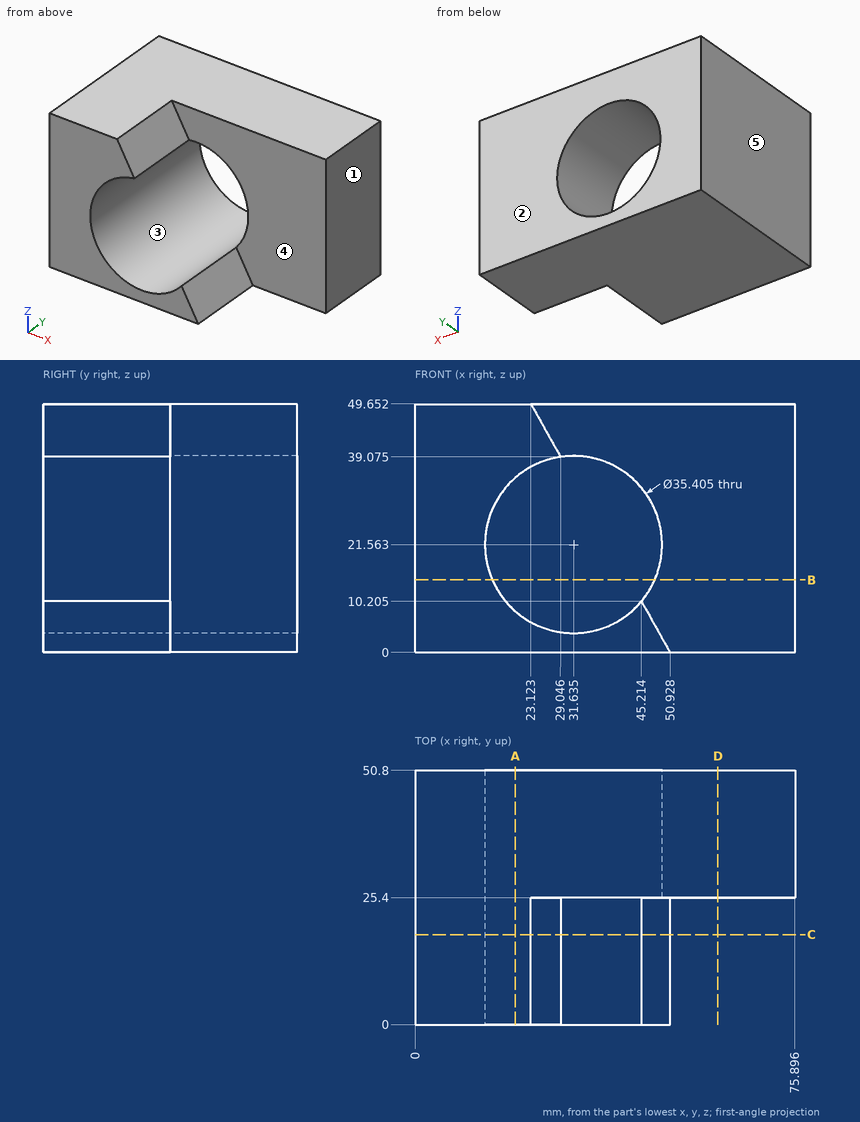
Verification items for this drawing (mm, ordinates from the low corner). A direction names the side the tool comes from. Coordinates: 2 decimals unless noted, no trailing zeros. Loops run counter-clockwise (first coordinate to the right, second up) from the corner with the lowest first, then second, coordinate; pieces in that order, holes last. Notation, with made-up numbers: (-9.75, 38) - (11.25, 38) arc R4 cw to (11.25, 44) - close; hole circle Ø10 at (46.25, -13.75). An arc over 180 degrees is marked (long way). Answer as a JSON object with one key per item and string values.
(1) Scan lines: line 1 along X through (y, z) = (47.5, 21); line 2 along X through (y, z) = (9, 21); line 3 along X through (y, z) = (40, 5.5) (1 decimal). Record each from-to range of solid material in increasing order.
Response:
{"line 1": "x = 0 to 13.94, 49.33 to 75.9", "line 2": "x = 0 to 13.94", "line 3": "x = 0 to 24.2, 39.1 to 75.9"}
(2) Go/stop test with flat-tipped pins: pin 1 Ø2 at (y, z) = (27.5, 11) entering from -X; pin 2 Ø2 at (y, z) = (11, 28) entering from +X; pin 3 Ø2 at (x, z) = (50.5, 12) entering from -Y. Record where each tip stops, or that it passes through.
Response:
{"pin 1": "stops at x = 0", "pin 2": "stops at x = 15.57", "pin 3": "stops at y = 25.4"}
(3) Cross-section at B-B, the plane z = 14.5. Record the boundary of the cut face in (x, y).
Response:
{"outline": "(0, 0) - (15.4, 0) - (15.4, 50.8) - (0, 50.8) - close; (47.87, 25.4) - (75.9, 25.4) - (75.9, 50.8) - (47.87, 50.8) - close"}
(4) Cross-section at D-D, the plane x = 60.5. Record the boundary of the cut face in (y, z).
Response:
{"outline": "(25.4, 0) - (50.8, 0) - (50.8, 49.65) - (25.4, 49.65) - close"}
(5) Mould release check, pull along X, two halves, no side actions. Record for the marked faces 1, 2 and 3: pulls with the +X half, pulls with the -X half, needs draft (parallel to the pull), parting line crosses it, or undercut.
Response:
{"face 1": "pulls with the +X half", "face 2": "needs draft", "face 3": "undercut"}
(6) Cross-section at C-C, the plane y = 18. Record the boundary of the cut face in (x, z) (1 decimal).
Response:
{"outline": "(0, 0) - (50.9, 0) - (45.2, 10.2) arc R17.7 cw (long way) to (29, 39.1) - (23.1, 49.7) - (0, 49.7) - close"}
(7) Access from +Z, -Z, +X, -X, +Y, -Y to the whole of each face (thin tool, end or side, straight path). Record for the marked faces 4 and 5.
Response:
{"face 4": "+Z, +X, -Y", "face 5": "+Z, -Z, -X, +Y, -Y"}
(8) Cross-section at A-A, the plane x = 20. Record the boundary of the cut face in (y, z) (1 decimal), then the cut area to 3 significant figures.
Response:
{"outline": "(0, 0) - (50.8, 0) - (50.8, 8.2) - (0, 8.2) - close; (0, 34.9) - (50.8, 34.9) - (50.8, 49.7) - (0, 49.7) - close", "area": "1,170 mm²"}
